Could you check a few things on this model? Use its own coordinates, in mm. Coordinates: 2 decimals unless noted, no trailing zeros. Loops run counter-clockwise (first coordinate to the right, second up) from the corner with the lowest first, then second, coordinate; pieces in that order, holes last.
1) Will these pins go through, and if not, where does the flat tip stop? P1, Ø5, axis at x = -10, y = -38, coming from the +Z side; P2, Ø6, axis at x = -4.5, z = -23.5, coming from the -Y side; P3, Ø6, axis at x = -9, y = 101.5, coming from the -Z side.
2) If I drill on line 1 along Z through (x, y) = (0, 171.5); line 2 along Z through (x, y) = (-12, 89); line 3 along X through (y, z) = (-13, 1), over which ranges is the centre line in solid material (lowest first)?
3) Imagine slicing it at A-A on y = 78. Please give me the cut outline in (x, z).
4) Thinking about a two-plate mould opening in X: for faces 1 (the face through (15, 200, -3)), 2 (the face through (-14.985, 101.642, 0.66)), 3 (the face through (-4.336, 101.642, -19.524)), which applies, released by +X, released by -X, zero draft, split by the parting line, or undercut?
```python
from build123d import *

# Parameters (mm, degrees)
F2_R   = 20
F2_R_2 = 15


with BuildPart() as f3:
    # F3: sweep along a path in F0
    with BuildLine(Plane.YZ) as f3_path:
        Line((200, 0), (6.000288, 0))
        ThreePointArc((6.000288, 0), (0.253077, -0.84355), (-5.009327, -3.303043))
        Line((-5.009327, -3.303043), (-83.484786, -55.048074))
    # F2 (on offset) → F3 (sweep)
    with BuildSketch(Plane.XZ.offset(-200)):
        Circle(F2_R)
        Circle(F2_R_2, mode=Mode.SUBTRACT)
    sweep(path=f3_path.line)


solid = f3.part
```
Filled in:
1. P1: stops at z = -2.05
1. P2: stops at y = -75.73
1. P3: stops at z = -19.08
2. line 1: z = -20 to -15, 15 to 20
2. line 2: z = -16 to -9, 9 to 16
2. line 3: x = -18.33 to -12.69, 12.69 to 18.33
3. outline: circle Ø40 at (0, 0); hole circle Ø30 at (0, 0)
4. face 1: zero draft
4. face 2: undercut
4. face 3: split by the parting line
